Can you work these out from the model? Positions are in its coordinate system, mm. Face numbers are marked on the shaded views. A direction names the side the tool comes from. Coordinates: 2 decimals unless noted, no trailing zeros. Order: outer loops, then holes, each group sorted by start corner. A loop starts at its lowest first (then second) coordinate and runs counter-clockwise, first axis right, second up. Notation, with made-up numbers: M 17,24.25 L 24,24.25 A15 cw 24,29.25 Z; hole C -26.5,22 d5. An arc over 180 degrees is marked long. Answer as a JSON object with one key per item and string values.
from build123d import *

# Parameters (mm, degrees)
EXTRUDE_1_DEPTH     = 10
FILLET_1_R          = 10
SHELL_1_T           = -2
SKETCH_2_R          = 7.5
CUT_EXTRUDE_1_DEPTH = 10
FILLET_2_R          = 1


with BuildPart() as part:
    # 草图1 → 凸台-拉伸1 (new body)
    with BuildSketch(Plane.XY):
        with BuildLine():
            add(Edge.make_bspline(
                [(-18.059479814, 8.593904168), (-23.948193256, -3.780809287), (-29.696472288, -24.34126392), (-30, -45.953108691), (-30, -54.460180984)],
                knots=[0, 0, 0, 0, 0.608662134, 1, 1, 1, 1], degree=3))
            Line((-30, -54.460180984), (-30, -64.460180984))
            ThreePointArc((-30, -64.460180984), (0, -70), (30, -64.460180984))
            Line((30, -64.460180984), (30, -54.460180984))
            add(Edge.make_bspline(
                [(18.059479814, 8.593904168), (23.423782854, -2.678798038), (29.865056496, -24.432184966), (30, -46.291744963), (30, -54.460180984)],
                knots=[0, 0, 0, 0, 0.608662134, 1, 1, 1, 1], degree=3))
            ThreePointArc((18.059479814, 8.593904168), (0, 20), (-18.059479814, 8.593904168))
        make_face()
    extrude(amount=EXTRUDE_1_DEPTH)

    # 圆角1
    fillet_1_edges = [part.edges().sort_by_distance(p)[0] for p in [
        (30, -64.460180984, 5),
        (-30, -64.460180984, 5),
    ]]
    fillet(fillet_1_edges, radius=FILLET_1_R)

    # 抽壳1
    shell_1_openings = [part.faces().sort_by_distance(p)[0] for p in [
        (0, -33.886417401, 0),
    ]]
    offset(amount=SHELL_1_T, openings=shell_1_openings, kind=Kind.INTERSECTION)

    # 草图2 → 切除-拉伸1 (cut)
    with BuildSketch(Plane.XY.offset(10)):
        Circle(SKETCH_2_R)
        with Locations((0, -45)):
            Circle(SKETCH_2_R)
    extrude(amount=-CUT_EXTRUDE_1_DEPTH, mode=Mode.SUBTRACT)

    # 圆角2
    fillet_2_edges = [part.edges().sort_by_distance(p)[0] for p in [
        (-30, -55.853116753, 10),
        (0, -70, 10),
        (30, -55.853116753, 10),
        (27.969536593, -63.286457019, 10),
        (-27.969536593, -63.286457019, 10),
        (-7.5, 0, 10),
        (-7.5, -45, 10),
        (0, 20, 10),
    ]]
    fillet(fillet_2_edges, radius=FILLET_2_R)


solid = part.part
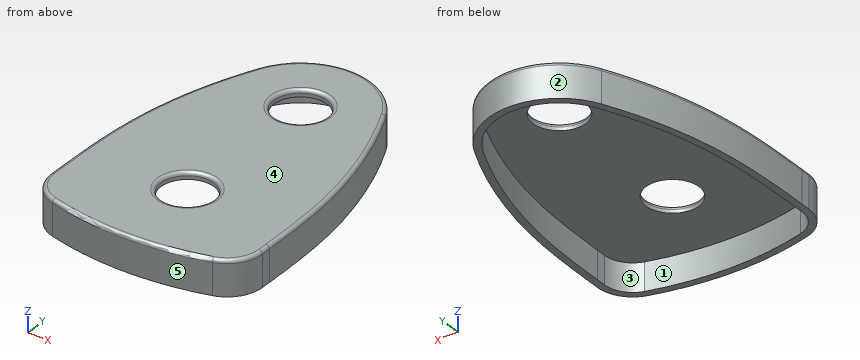
Item 1: I want a section at A-A, the plane x = 0. Write out the boundary of the cut face in (y, z), plus the area to 3 significant figures.
Answers follow:
{"outline": "M -70,0 L -68,0 L -68,8 L -52.5,8 L -52.5,9 A1 ccw -53.5,10 L -69,10 A1 ccw -70,9 Z; M -37.5,8 L -7.5,8 L -7.5,9 A1 ccw -8.5,10 L -36.5,10 A1 ccw -37.5,9 Z; M 7.5,8 L 18,8 L 18,0 L 20,0 L 20,9 A1 ccw 19,10 L 8.5,10 A1 ccw 7.5,9 Z", "area": "151 mm^2"}
Item 2: I'm going to push flat-ended pins straight in: pin 1 (9 mm diameter, centred on x = 0, y = -45, fed in from +Z); pin 2 (17 mm diameter, centred on x = -5, y = -36.5, fed in from -Z); pin 3 (6 mm diameter, centred on y = -15, z = 6, fed in from +X); pin 4 (6 mm diameter, centred on y = -12.5, z = 4, fed in from -X). Where does each tip first touch, or does it pass through?
Answers follow:
{"pin 1": "passes through", "pin 2": "stops at z = 8", "pin 3": "stops at x = 27.05", "pin 4": "stops at x = -26.55"}
Item 3: Which directions (+Z, -Z, +X, -X, +Y, -Y) give clear straight access to the entire face, cutting with the end or side of a thin tool? Please do the marked faces 1 and 2.
Answers follow:
{"face 1": "-Z", "face 2": "+Z, -Z, +Y"}
Item 4: If we mould it in two halves opening along Y, with no side actions, what happens to the marked faces 3, 4 and 5? For each: pulls with the +Y half, pulls with the -Y half, needs draft (parallel to the pull), parting line crosses it, or undercut.
Answers follow:
{"face 3": "undercut", "face 4": "needs draft", "face 5": "pulls with the -Y half"}
Item 5: Please list where these lines run through material, in increasing order: line 1 (X direction, y = -52.5, z = 7.25); line 2 (Z direction, x = 10, y = 5); line 3 (Y direction, x = -3.5, z = 5.5).
Answers follow:
{"line 1": "x = -30 to -28, 28 to 30", "line 2": "z = 8 to 10", "line 3": "y = -69.93 to -67.93, 17.66 to 19.69"}
